Read the model definition and answer for the solid it produces. Units are mm, in the model's axes. A direction names the side the tool comes from. Coordinates: 2 decimals unless noted, no trailing zeros. Loops run counter-clockwise (first coordinate to the right, second up) from the corner with the lowest first, then second, coordinate; pieces in that order, holes last. Notation, with made-up numbers: (21, 61) - (54, 61) arc R21 ccw to (54, 95) - close; hole circle Ø6 at (-12, 70.25). An arc over 180 degrees is marked (long way). Use one line per item in the form item = value.
from build123d import *

# Parameters (mm, degrees)
SKETCH1_R      = 2.5
EXTRUDE1_DEPTH = 13
EXTRUDE2_DEPTH = 8
EXTRUDE3_START = 20
EXTRUDE3_DEPTH = 20
FILLET1_R      = 10
FILLET2_R      = 10
SKETCH4_R      = 2.5
EXTRUDE4_DEPTH = 113.911387675


with BuildPart() as part:
    # Sketch1 → Extrude1 (new body)
    with BuildSketch(Plane.XY):
        with BuildLine():
            Line((-9, 56.394324189), (-9, -98.605675811))
            ThreePointArc((-9, -98.605675811), (0, -107.605675811), (9, -98.605675811))
            Line((9, -98.605675811), (9, 56.394324189))
            ThreePointArc((9, 56.394324189), (0, 65.394324189), (-9, 56.394324189))
        make_face()
        with Locations(Location((0, 56.394324189, 0), (0, 0, 180))):
            Circle(SKETCH1_R, mode=Mode.SUBTRACT)
        with Locations(Location((0, -98.605675811, 0), (0, 0, 180))):
            Circle(SKETCH1_R, mode=Mode.SUBTRACT)
    extrude(amount=EXTRUDE1_DEPTH)

    # Sketch2 → Extrude2 (cut)
    with BuildSketch(Plane.XY.offset(13)):
        with BuildLine():
            Line((-5, -3.605675811), (-5, -83.605675811))
            ThreePointArc((-5, -83.605675811), (0, -88.605675811), (5, -83.605675811))
            Line((5, -83.605675811), (5, -3.605675811))
            ThreePointArc((5, -3.605675811), (0, 1.394324189), (-5, -3.605675811))
        make_face()
    extrude(amount=-EXTRUDE2_DEPTH, mode=Mode.SUBTRACT)

    # Sketch3 → Extrude3 (add)
    with BuildSketch(Plane(origin=(0, 0, 0), x_dir=(-1, 0, 0), z_dir=(0, 0, -1)).offset(EXTRUDE3_START)):
        with BuildLine():
            Line((-9, 56.394324189), (-9, 24.585637313))
            Line((-9, 24.585637313), (9, 24.585637313))
            Line((9, 24.585637313), (9, 56.394324189))
            ThreePointArc((9, 56.394324189), (0, 65.394324189), (-9, 56.394324189))
        make_face()
    extrude(amount=-EXTRUDE3_DEPTH)

    # Fillet1
    fillet1_edges = [part.edges().sort_by_distance(p)[0] for p in [
        (9, 24.585637313, -10),
    ]]
    fillet(fillet1_edges, radius=FILLET1_R)

    # Fillet2
    # the kernel refuses this fillet: 10 mm, written as the material it takes off along each edge
    with BuildSketch(Plane(origin=(-9, 24.585637313, -44.494897428), x_dir=(0, 1, 0), z_dir=(0, 0, 1))) as fillet2_piece_1:
        with BuildLine():
            CenterArc((9.797958971, -10), FILLET2_R, 90, 78.463040967)
            Line((0, -8), (-0.195959179, -7.96))
            ThreePointArc((-0.195959179, -7.96), (-0.2, -4), (-0.2, 0))
            Line((-0.2, 0), (0, 0.2))
            Line((0, 0.2), (9.797958971, 0.2))
            Line((9.797958971, 0.2), (9.797958971, 0))
        make_face()
    extrude(amount=44.494897428, mode=Mode.SUBTRACT)

    # Sketch4 → Extrude4 (cut, through all)
    with BuildSketch(Plane.XY.offset(13)):
        with Locations(Location((0, 56.394324189, 0), (0, 0, 180))):
            Circle(SKETCH4_R)
    extrude(amount=-EXTRUDE4_DEPTH, mode=Mode.SUBTRACT)


solid = part.part
Item 1: Which of the six approach directions +Z, -Z, +X, -X, +Y, -Y give full straight-line access (tool end or side, diameter ignored) to faces 1 (the cylindrical face through (-6.806, 28.134, -10.14)), 2 (the cylindrical face through (-0.198, -107.603, 6.409)), 3 (the cylindrical face through (-0.11, -88.604, 9.056)), 4 (the cylindrical face through (6.148, 27.593, -9.86)), 5 (the flat face through (0, 45, -20))?
Results below:
face_1 = -Z, -X, -Y
face_2 = +Z, -Z, -Y
face_3 = +Z
face_4 = -Z, +X, -Y
face_5 = -Z, +X, -X, +Y, -Y
Item 2: The part is cut by section C-C on x = 0.75. Give the vertices of the cut face in (y, z).
Results below:
outline = (-107.57, 0) - (-100.99, 0) - (-100.99, 13) - (-107.57, 13) - close; (-96.22, 0) - (24.74, 0) - (24.74, -20) - (54.01, -20) - (54.01, 13) - (1.34, 13) - (1.34, 5) - (-88.55, 5) - (-88.55, 13) - (-96.22, 13) - close; (58.78, -20) - (65.36, -20) - (65.36, 13) - (58.78, 13) - close
Item 3: The part is cut by section B-B on z = -8. Give the vertices of the cut face in (x, y).
Results below:
outline = (-9, 34.38) arc R10 ccw to (-1, 24.59) arc R10 ccw to (9, 34.59) - (9, 56.39) arc R9 ccw to (-9, 56.39) - close; hole circle Ø5 at (0, 56.39)
Item 4: The part is cut by section A-A on z = 8. Give the vertices of the cut face in (x, y), plus the area to 3 significant figures.
Results below:
outline = (-9, -98.61) arc R9 ccw to (9, -98.61) - (9, 56.39) arc R9 ccw to (-9, 56.39) - close; hole (-5, -83.61) arc R5 ccw to (5, -83.61) - (5, -3.61) arc R5 ccw to (-5, -3.61) - close; hole circle Ø5 at (0, -98.61); hole circle Ø5 at (0, 56.39)
area = 2,130 mm²
Item 5: Each of these flat-tipped pins is pushed along its axis until it touches: P1, Ø3, axis at x = 7, y = -90, coming from the -Z side; P2, Ø1.5, axis at x = -1, y = -18, coming from the +Z side; P3, Ø4, axis at x = 0, y = -98.61, coming from the -Z side; P4, Ø8, axis at x = -0.5, z = -15.5, coming from the -Y side. Where does it stop, or does it pass through?
Results below:
P1 = 0
P2 = 5
P3 = through
P4 = 24.59
Item 6: For a pull along X with two mould halves and no side action, classify faces 6 (the flat face through (-5, -43, 9)), 7 (the flat face through (-9, -5, 4)), 8 (the flat face through (9, -3, 4)) as +X half, -X half, draft (parallel to the pull), parting line (faces both ways), or undercut.
Results below:
face_6 = undercut
face_7 = -X half
face_8 = +X half
Item 7: The part is cut by section D-D on y = 29.5. Give the vertices of the cut face in (x, z), plus the area to 3 significant figures.
Results below:
outline = (-9, 0) - (-7.73, 0) - (-7.73, -20) - (7.61, -20) - (7.61, 0) - (9, 0) - (9, 13) - (-9, 13) - close
area = 541 mm²
Item 8: Find the intervals of material crossed by L1, parallel to Y at x = 0, z = 3.5; L2, parallel to X at y = -58.5, z = 8.5; L3, parallel to Z at x = 6, y = -81, in increasing order.
Results below:
L1 = -107.61 to -101.11, -96.11 to 53.89, 58.89 to 65.39
L2 = -9 to -5, 5 to 9
L3 = 0 to 13
